Read the model definition and answer for the solid it produces. Units are mm, in the model's axes. Face numbers are marked on the shaded views. A direction names the side the tool comes from. Coordinates: 2 decimals unless noted, no trailing zeros. Loops run counter-clockwise (first coordinate to the right, second up) from the corner with the lowest first, then second, coordinate; pieces in that order, holes last. Notation, with made-up numbers: (37, 88.25) - (80, 88.25) arc R32 ccw to (80, 120.25) - close; hole circle Ø8 at (65.5, -4.75). An arc over 180 degrees is marked (long way). Use one line per item in the form item = value. Start each with the question number.
1) Consider line 1 (X direction, y = 13.25, z = 27); line 2 (X direction, y = 26.4, z = 45); line 3 (X direction, y = 9.5, z = 16). Determine where each line is inside the solid, lowest interval first.
2) Each of these flat-tipped pins is pushed along its axis until it touches: P1, Ø1, axis at x = 13.5, y = 11.5, coming from the -Z side; P2, Ø3, axis at x = 91.5, z = -24.5, coming from the +Y side; P3, Ø5, axis at x = -52, y = 10.5, coming from the +Z side. Where does it stop, or does it pass through?
3) A cutting plane is placed at B-B (x = 66). Give the vertices of the cut face in (y, z), and give its area (3 significant figures).
4) The mould has two halves that part along X. Classify the marked faces 3, 4 and 5: released by +X, released by -X, zero draft, split by the parting line, or undercut.
5) Which of the six approach directions +Z, -Z, +X, -X, +Y, -Y give full straight-line access (tool end or side, diameter ignored) to the marked faces 1 and 2?
6) A cutting plane is placed at C-C (z = 14). Give the vertices of the cut face in (x, y).
7) A cutting plane is placed at A-A (z = -45). Give the vertices of the cut face in (x, y).
from build123d import *
from OCP.BRepFilletAPI import BRepFilletAPI_MakeChamfer

# Parameters (mm, degrees)
SKETCH_1_W          = 200
SKETCH_1_H          = 80
SKETCH_1_W_2        = 177
SKETCH_1_H_2        = 40
EXTRUDE_1_DEPTH     = 5
CHAMFER_1_SIZE      = 3
CHAMFER_1_SIZE2     = 1.732050808
SKETCH_2_W          = 200
SKETCH_2_H          = 80
EXTRUDE_2_DEPTH     = 2
SKETCH_3_W          = 200
SKETCH_3_H          = 80
SKETCH_3_R          = 1.25
EXTRUDE_3_DEPTH     = 10.5
SKETCH_4_W          = 200
SKETCH_4_H          = 80
SKETCH_4_W_2        = 192
SKETCH_4_H_2        = 65
EXTRUDE_4_DEPTH     = 10
CHAMFER_2_SIZE      = 5
SKETCH_6_W          = 16
SKETCH_6_H          = 10
SKETCH_6_R          = 2.1
EXTRUDE_6_DEPTH     = 5
EXTRUDE_9_DEPTH     = 16
EXTRUDE_10_DEPTH    = 16
SKETCH_12_W         = 10
SKETCH_12_H         = 10
CUT_EXTRUDE_2_DEPTH = 22
CHAMFER_3_SIZE      = 2
CHAMFER_3_SIZE2     = 3.464101615


with BuildPart() as part:
    # Эскиз1 → Бобышка-Вытянуть1 (new body)
    with BuildSketch(Plane(origin=(0, 0, 0), x_dir=(1, 0, 0), z_dir=(0, 1, 0))):
        Rectangle(SKETCH_1_W, SKETCH_1_H)
        Rectangle(SKETCH_1_W_2, SKETCH_1_H_2, mode=Mode.SUBTRACT)
    extrude(amount=EXTRUDE_1_DEPTH)

    # Фаска1
    chamfer_1_edges = [part.edges().sort_by_distance(p)[0] for p in [
        (0, 5, -20),
        (0, 5, 20),
    ]]
    chamfer_1_side = [part.faces().sort_by_distance(p)[0] for p in [
        (0, 5, -37.845934077),
    ]]
    chamfer(chamfer_1_edges, length=CHAMFER_1_SIZE, length2=CHAMFER_1_SIZE2, reference=chamfer_1_side[0])

    # Эскиз2 → Бобышка-Вытянуть2 (add)
    with BuildSketch(Plane(origin=(0, 5, 0), x_dir=(1, 0, 0), z_dir=(0, 1, 0))):
        Rectangle(SKETCH_2_W, SKETCH_2_H)
        Polygon((-88.5, 30), (-88.5, -28), (-48.5, -28), (-48.5, -32), (-32.5, -32), (-32.5, -28), (32.5, -28), (32.5, -32), (48.5, -32), (48.5, -28), (88.5, -28), (88.5, 30), (77, 30), (77, 23), (52.5, 23), (52.5, 30), (41.5, 30), (41.5, 23), (-41.5, 23), (-41.5, 30), (-52.5, 30), (-52.5, 23), (-77, 23), (-77, 30), align=None, mode=Mode.SUBTRACT)
    extrude(amount=EXTRUDE_2_DEPTH)

    # Эскиз3 → Бобышка-Вытянуть3 (add)
    with BuildSketch(Plane(origin=(0, 7, 0), x_dir=(1, 0, 0), z_dir=(0, 1, 0))):
        Rectangle(SKETCH_3_W, SKETCH_3_H)
        with Locations(Location((-91.5, 25, 0), (0, 0, 90))):
            Circle(SKETCH_3_R, mode=Mode.SUBTRACT)
        with Locations(Location((91.5, 25, 0), (0, 0, 90))):
            Circle(SKETCH_3_R, mode=Mode.SUBTRACT)
        with Locations(Location((-91.5, -27, 0), (0, 0, 90))):
            Circle(SKETCH_3_R, mode=Mode.SUBTRACT)
        with Locations(Location((91.5, -27, 0), (0, 0, 90))):
            Circle(SKETCH_3_R, mode=Mode.SUBTRACT)
        Polygon((-93, 22), (-88.5, 22), (-88.5, 30), (88.5, 30), (88.5, 22), (93, 22), (93, -19), (88.5, -19), (88.5, -33), (-88.5, -33), (-88.5, -19), (-93, -19), align=None, mode=Mode.SUBTRACT)
    extrude(amount=EXTRUDE_3_DEPTH)

    # Эскиз4 → Бобышка-Вытянуть4 (add)
    with BuildSketch(Plane(origin=(0, 17.5, 0), x_dir=(1, 0, 0), z_dir=(0, 1, 0))):
        Rectangle(SKETCH_4_W, SKETCH_4_H)
        with Locations((0, -0.5)):
            Rectangle(SKETCH_4_W_2, SKETCH_4_H_2, mode=Mode.SUBTRACT)
    extrude(amount=EXTRUDE_4_DEPTH)

    # Фаска2
    chamfer_2_edges = [part.edges().sort_by_distance(p)[0] for p in [
        (0, 0, -40),
        (100, 0, 0),
        (0, 0, 40),
        (-100, 0, 0),
    ]]
    chamfer(chamfer_2_edges, length=CHAMFER_2_SIZE)

    # Эскиз6 → Бобышка-Вытянуть6 (add)
    # profile 1 of 4: a face of its own
    with BuildSketch(Plane(origin=(0, 27.5, 0), x_dir=(1, 0, 0), z_dir=(0, 1, 0))):
        with Locations((-92, 45)):
            Rectangle(SKETCH_6_W, SKETCH_6_H)
        with Locations(Location((-92, 45, 0), (0, 0, 270))):
            Circle(SKETCH_6_R, mode=Mode.SUBTRACT)
    # profile 2 of 4: a face of its own
    with BuildSketch(Plane(origin=(0, 27.5, 0), x_dir=(1, 0, 0), z_dir=(0, 1, 0))):
        with Locations((92, 45)):
            Rectangle(SKETCH_6_W, SKETCH_6_H)
        with Locations(Location((92, 45, 0), (0, 0, 270))):
            Circle(SKETCH_6_R, mode=Mode.SUBTRACT)
    # profile 3 of 4: a face of its own
    with BuildSketch(Plane(origin=(0, 27.5, 0), x_dir=(1, 0, 0), z_dir=(0, 1, 0))):
        with Locations((92, -45)):
            Rectangle(SKETCH_6_W, SKETCH_6_H)
        with Locations(Location((92, -45, 0), (0, 0, 270))):
            Circle(SKETCH_6_R, mode=Mode.SUBTRACT)
    # profile 4 of 4: a face of its own
    with BuildSketch(Plane(origin=(0, 27.5, 0), x_dir=(1, 0, 0), z_dir=(0, 1, 0))):
        with Locations((-92, -45)):
            Rectangle(SKETCH_6_W, SKETCH_6_H)
        with Locations(Location((-92, -45, 0), (0, 0, 270))):
            Circle(SKETCH_6_R, mode=Mode.SUBTRACT)
    extrude(amount=-EXTRUDE_6_DEPTH)

    # Эскиз10 → Бобышка-Вытянуть9 (add)
    with BuildSketch(Plane(origin=(100, 0, 0), x_dir=(0, 0, -1), z_dir=(1, 0, 0))):
        Polygon((-50, 22.5), (-40, 5), (-40, 22.5), align=None)
        Polygon((40, 5), (50, 22.5), (40, 22.5), align=None)
    extrude(amount=-EXTRUDE_9_DEPTH)

    # Эскиз11 → Бобышка-Вытянуть10 (add)
    with BuildSketch(Plane.ZY.offset(100)):
        Polygon((-50, 22.5), (-40, 22.5), (-40, 5), align=None)
        Polygon((40, 5), (50, 22.5), (40, 22.5), align=None)
    extrude(amount=-EXTRUDE_10_DEPTH)

    # Эскиз12 → Вырез-Вытянуть2 (cut)
    with BuildSketch(Plane(origin=(0, 22.5, 0), x_dir=(1, 0, 0), z_dir=(0, 1, 0))):
        with Locations((-92, -45)):
            Rectangle(SKETCH_12_W, SKETCH_12_H)
        with Locations((-92, 45)):
            Rectangle(SKETCH_12_W, SKETCH_12_H)
        with Locations((92, 45)):
            Rectangle(SKETCH_12_W, SKETCH_12_H)
        with Locations((92, -45)):
            Rectangle(SKETCH_12_W, SKETCH_12_H)
    extrude(amount=-CUT_EXTRUDE_2_DEPTH, mode=Mode.SUBTRACT)

    # Фаска3: one chamfer whose edges measure the first distance from different faces: ONE call of the kernel's chamfer builder (chamfer() names one face for all edges)
    chamfer_3_edges_1 = [part.edges().sort_by_distance(p)[0] for p in [
        (88.5, 0, 0),
    ]]
    chamfer_3_side_1 = [part.faces().sort_by_distance(p)[0] for p in [
        (88.5, 1.633974596, -19.346146041),
    ]]
    chamfer_3_edges_2 = [part.edges().sort_by_distance(p)[0] for p in [
        (0, 0, -20),
    ]]
    chamfer_3_side_2 = [part.faces().sort_by_distance(p)[0] for p in [
        (0, 1.633974596, -20),
    ]]
    chamfer_3_edges_3 = [part.edges().sort_by_distance(p)[0] for p in [
        (-88.5, 0, 0),
    ]]
    chamfer_3_side_3 = [part.faces().sort_by_distance(p)[0] for p in [
        (-88.5, 1.633974596, 19.346146041),
    ]]
    chamfer_3_edges_4 = [part.edges().sort_by_distance(p)[0] for p in [
        (0, 0, 20),
    ]]
    chamfer_3_side_4 = [part.faces().sort_by_distance(p)[0] for p in [
        (0, 1.633974596, 20),
    ]]
    chamfer_3 = BRepFilletAPI_MakeChamfer(part.part.solid().wrapped)
    for e in chamfer_3_edges_1:
        chamfer_3.Add(CHAMFER_3_SIZE, CHAMFER_3_SIZE2, e.wrapped, chamfer_3_side_1[0].wrapped)  # the first distance lies on this face
    for e in chamfer_3_edges_2:
        chamfer_3.Add(CHAMFER_3_SIZE, CHAMFER_3_SIZE2, e.wrapped, chamfer_3_side_2[0].wrapped)  # the first distance lies on this face
    for e in chamfer_3_edges_3:
        chamfer_3.Add(CHAMFER_3_SIZE, CHAMFER_3_SIZE2, e.wrapped, chamfer_3_side_3[0].wrapped)  # the first distance lies on this face
    for e in chamfer_3_edges_4:
        chamfer_3.Add(CHAMFER_3_SIZE, CHAMFER_3_SIZE2, e.wrapped, chamfer_3_side_4[0].wrapped)  # the first distance lies on this face
    add(Compound.cast(chamfer_3.Shape()), mode=Mode.REPLACE)


solid = part.part
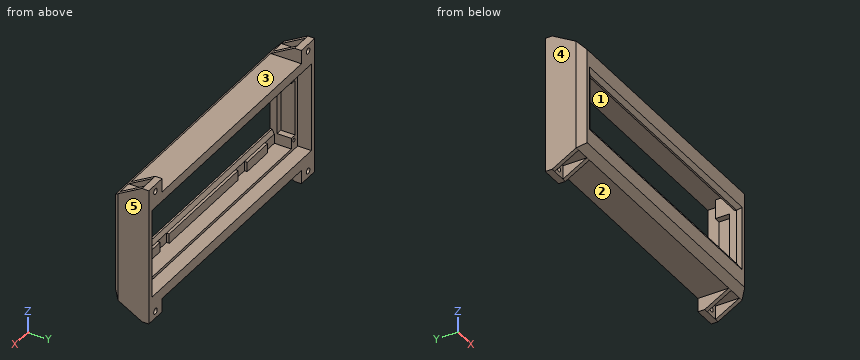
Found:
q1.line_1 = -100 to -92.75, -90.25 to -88.5, 88.5 to 90.25, 92.75 to 100
q1.line_2 = -100 to -94.1, -89.9 to -84, 84 to 89.9, 94.1 to 100
q1.line_3 = -100 to -93, 93 to 100
q2.P1 = -40
q2.P2 = 17.5
q2.P3 = 40
q3.outline = (0, -35) - (5, -40) - (27.5, -40) - (27.5, -32) - (17.5, -32) - (17.5, -30) - (7, -30) - (7, -23) - (5, -23) - (3.27, -20) - (2, -20) - (0, -23.46) - close; (0, 23.46) - (2, 20) - (3.27, 20) - (5, 23) - (5, 28) - (7, 28) - (7, 33) - (27.5, 33) - (27.5, 40) - (5, 40) - (0, 35) - close
q3.area = 549 mm^2
q4.face_3 = undercut
q4.face_4 = released by -X
q4.face_5 = released by +X
q5.face_1 = +Y
q5.face_2 = -Z, +Y, -Y
q6.outline = (-100, 5) - (-95, 0) - (-91.96, 0) - (-88.5, 2) - (-88.5, 7) - (-93, 7) - (-93, 17.5) - (-96, 17.5) - (-96, 27.5) - (-100, 27.5) - close; (88.5, 2) - (91.96, 0) - (95, 0) - (100, 5) - (100, 27.5) - (96, 27.5) - (96, 17.5) - (93, 17.5) - (93, 7) - (88.5, 7) - close
q7.outline = (-100, 13.75) - (-97, 13.75) - (-97, 22.5) - (-94.1, 22.5) - (-94.1, 27.5) - (-100, 27.5) - close; (-89.9, 22.5) - (-87, 22.5) - (-87, 13.75) - (-84, 13.75) - (-84, 27.5) - (-89.9, 27.5) - close; (84, 13.75) - (87, 13.75) - (87, 22.5) - (89.9, 22.5) - (89.9, 27.5) - (84, 27.5) - close; (94.1, 22.5) - (97, 22.5) - (97, 13.75) - (100, 13.75) - (100, 27.5) - (94.1, 27.5) - close
